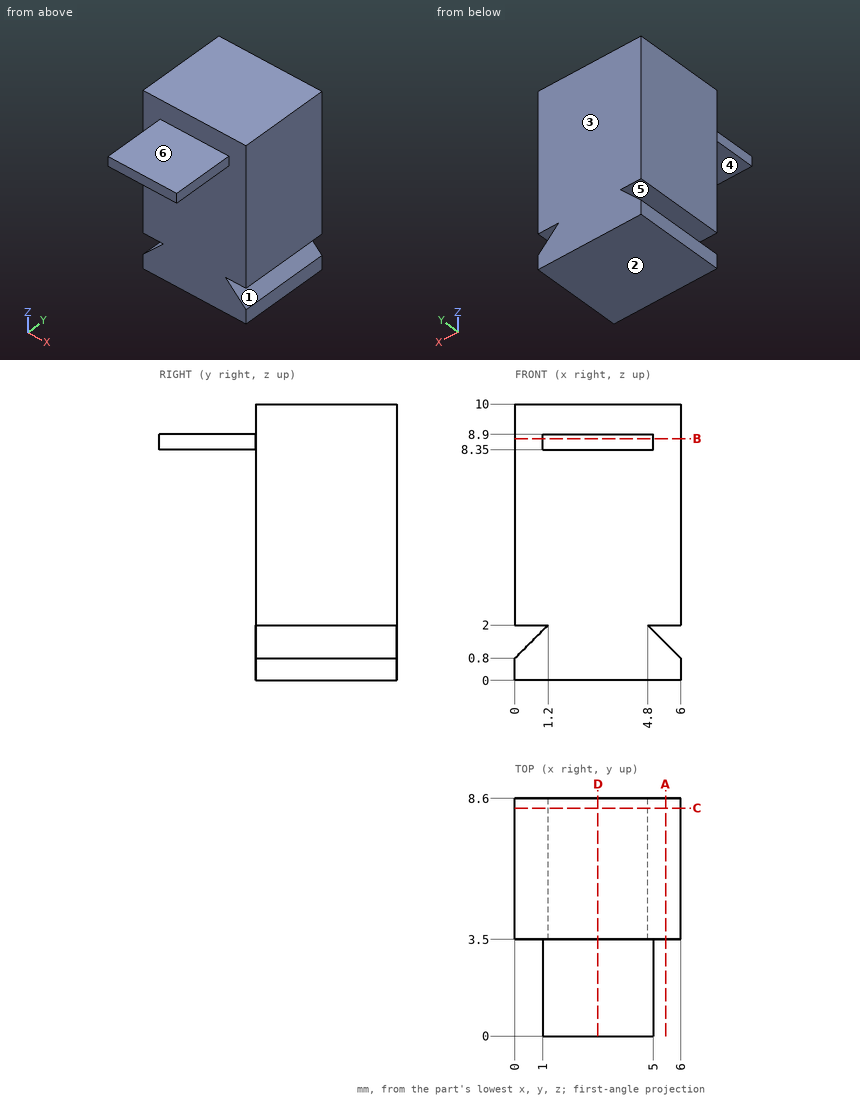
For this review, use the dimensioned drawing (mm, ordinates from the lowest corner) and the shaded views. A direction names the side the tool comes from. Round coordinates to 2 decimals unless told otherwise and drop trailing zeros. Write each loop counter-clockwise with the first axis right and the second up, starting at its lowest first coordinate (ties: lowest second). Pieces come first, ordered by that corner, then holes. Notation, with made-up numbers: (19.5, -19.75) - (39.5, -19.75) arc R18 cw to (39.5, -9.75) - close; hole circle Ø9 at (60.25, 12.5). An arc over 180 degrees is marked (long way). Use a Markdown table: item, result.
Q1. The part is to be moulded in two halves that separate along Z. For the marked faces 3, 4, 5 and 6, say which applies: pulls with the +Z half, pulls with the -Z half, needs draft (parallel to the pull), parting line crosses it, or undercut.
Derived:
| item | result |
|---|---|
| face 3 | needs draft |
| face 4 | pulls with the -Z half |
| face 5 | undercut |
| face 6 | pulls with the +Z half |
Q2. We need section B-B (z = 8.75). Give the boundary of the cut face in (x, y).
Derived:
| item | result |
|---|---|
| outline | (0, 3.5) - (1, 3.5) - (1, 0) - (5, 0) - (5, 3.5) - (6, 3.5) - (6, 8.6) - (0, 8.6) - close |
Q3. We need section C-C (y = 8.25). Give the boundary of the cut face in (x, z), plus the area to 3 significant figures.
Derived:
| item | result |
|---|---|
| outline | (0, 0) - (6, 0) - (6, 0.8) - (4.8, 2) - (6, 2) - (6, 10) - (0, 10) - (0, 2) - (1.2, 2) - (0, 0.8) - close |
| area | 58.6 mm2 |
Q4. We need section D-D (x = 3). Give the boundary of the cut face in (y, z).
Derived:
| item | result |
|---|---|
| outline | (0, 8.35) - (3.5, 8.35) - (3.5, 0) - (8.6, 0) - (8.6, 10) - (3.5, 10) - (3.5, 8.9) - (0, 8.9) - close |
Q5. Clearance check with a flat-ended pin moving along its axis: pin 1 (3 mm diameter, centred on x = 4.5, y = 1, fed in from -Z). State where the tip first meets the part, or that it passes through.
Derived:
| item | result |
|---|---|
| pin 1 | stops at z = 8.35 |
Q6. We need section A-A (x = 5.45). Give the boundary of the cut face in (y, z), plus the area to 3 significant figures.
Derived:
| item | result |
|---|---|
| outline | (3.5, 0) - (8.6, 0) - (8.6, 1.35) - (3.5, 1.35) - close; (3.5, 2) - (8.6, 2) - (8.6, 10) - (3.5, 10) - close |
| area | 47.7 mm2 |
Q7. Wall thickness on line 1 along Y through (x, z) = (1.45, 8); line 2 along Z through (x, y) = (2.1, 1); line 3 along Z through (x, y) = (1, 5): over which ranges is each line inside the solid? List them lowest first.
Derived:
| item | result |
|---|---|
| line 1 | y = 3.5 to 8.6 |
| line 2 | z = 8.35 to 8.9 |
| line 3 | z = 0 to 1.8, 2 to 10 |
Q8. Machinability: for the marked faces 1 and 2, which of the approach directions +Z, -Z, +X, -X, +Y, -Y give a long, thin tool a straight path to every point of the face, cutting with its end or side? Answer none if there is none.
Derived:
| item | result |
|---|---|
| face 1 | +X, +Y, -Y |
| face 2 | -Z, +X, -X, +Y, -Y |
